Design review of the part built by this model. Coordinates are the model's own, in mm. Give positions to 0.01 mm unless a question says otherwise; leave off trailing zeros. Loops run counter-clockwise (first coordinate to the right, second up) from the corner with the lowest first, then second, coordinate; pieces in that order, holes last. Notation, with made-up numbers: (20.5, -36.75) -> (61.5, -36.75) arc R9 cw to (61.5, -31.75) -> close; hole circle Ø8 at (38, 23). An arc over 180 degrees is marked (long way). Answer in a Markdown table with one row per item. Add a question column.
(1) Consider section A-A on x = -46. Write out the cut boundary in (y, z).
(2) For pin 1 (1 mm diameter, centred on x = 35, y = -4.5, fed in from -Z); pin 2 (2 mm diameter, centred on y = -30, z = 1, fed in from +X); pin 3 (2 mm diameter, centred on x = -55.5, z = 3, fed in from -Y); pin 4 (1.2 mm diameter, centred on x = 49, z = 1.5, fed in from +Y), all flat-tipped, find the tip position at first contact; note any pin that passes through.
(3) Consider section C-C on y = -7. Write out the cut boundary in (x, z), then the cut area to 3 significant figures.
(4) For line 1 (Y direction, x = -42.5, z = 0.4); line 2 (X direction, y = -16, z = 2.25); line 3 (X direction, y = 29, z = 1), list the stretches that pass through material, from the lowest coordinate up.
(5) Consider section B-B on z = 1.6. Write out the cut boundary in (x, y).
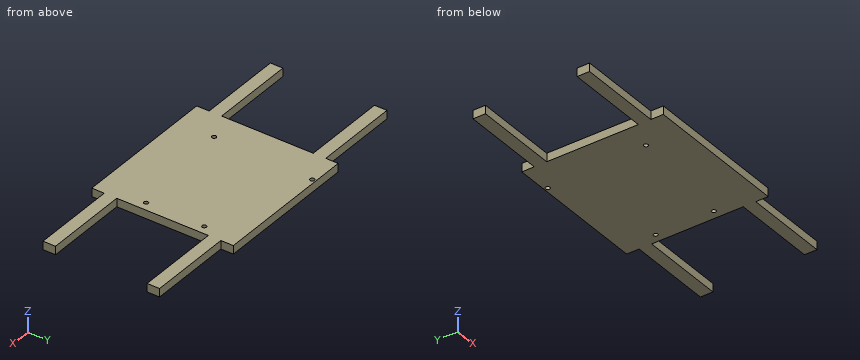
from build123d import *

# Parameters (mm, degrees)
SKETCH1_W           = 70
SKETCH1_H           = 68
SKETCH1_R           = 1.0287
BOSS_EXTRUDE1_DEPTH = 4
SKETCH2_W           = 40.88
SKETCH2_H           = 6
BOSS_EXTRUDE2_DEPTH = 4


with BuildPart() as part:
    # Sketch1 → Boss-Extrude1 (new body)
    with BuildSketch(Plane.XY):
        Rectangle(SKETCH1_W, SKETCH1_H)
        with Locations((-21.606472839, -15.978304245)):
            Circle(SKETCH1_R, mode=Mode.SUBTRACT)
        with Locations((30.793527161, -10.878304245)):
            Circle(SKETCH1_R, mode=Mode.SUBTRACT)
        with Locations((30.793527161, 17.021695755)):
            Circle(SKETCH1_R, mode=Mode.SUBTRACT)
        with Locations((-20.006472839, 32.321695755)):
            Circle(SKETCH1_R, mode=Mode.SUBTRACT)
    extrude(amount=BOSS_EXTRUDE1_DEPTH)

    # Sketch2 → Boss-Extrude2 (add)
    with BuildSketch(Plane(origin=(0, 0, 0), x_dir=(-1, 0, 0), z_dir=(0, 0, -1))):
        with Locations((55.44, 25)):
            Rectangle(SKETCH2_W, SKETCH2_H)
        with Locations((-55.44, 25)):
            Rectangle(SKETCH2_W, SKETCH2_H)
        with Locations((-55.44, -25)):
            Rectangle(SKETCH2_W, SKETCH2_H)
        with Locations((55.44, -25)):
            Rectangle(SKETCH2_W, SKETCH2_H)
    extrude(amount=-BOSS_EXTRUDE2_DEPTH)


solid = part.part
Values follow:
| question | item | result |
|---|---|---|
| 1 | outline | (-28, 0) -> (-22, 0) -> (-22, 4) -> (-28, 4) -> close; (22, 0) -> (28, 0) -> (28, 4) -> (22, 4) -> close |
| 2 | pin 1 | z = 0 |
| 2 | pin 2 | x = 35 |
| 2 | pin 3 | y = -28 |
| 2 | pin 4 | y = 28 |
| 3 | outline | (-35, 0) -> (35, 0) -> (35, 4) -> (-35, 4) -> close |
| 3 | area | 280 mm2 |
| 4 | line 1 | -28 to -22, 22 to 28 |
| 4 | line 2 | -35 to -22.63, -20.58 to 35 |
| 4 | line 3 | -35 to 35 |
| 5 | outline | (-75.88, -28) -> (-35, -28) -> (-35, -34) -> (35, -34) -> (35, -28) -> (75.88, -28) -> (75.88, -22) -> (35, -22) -> (35, 22) -> (75.88, 22) -> (75.88, 28) -> (35, 28) -> (35, 34) -> (-35, 34) -> (-35, 28) -> (-75.88, 28) -> (-75.88, 22) -> (-35, 22) -> (-35, -22) -> (-75.88, -22) -> close; hole circle Ø2.06 at (-21.61, -15.98); hole circle Ø2.06 at (-20.01, 32.32); hole circle Ø2.06 at (30.79, -10.88); hole circle Ø2.06 at (30.79, 17.02) |
